The listing builds one solid part. Answer for the finished solid, in the listing's coordinates (mm). Give positions to 0.01 mm unless a question says otherwise; leave off trailing zeros. Order: outer loops, then holes, each group sorted by start corner. A loop starts at its lowest first (then second) coordinate and runs counter-clockwise, first axis right, second up. Notation, with made-up numbers: (1.5, 25.5) - (25.5, 25.5) arc R27 cw to (25.5, 57.5) - close; hole circle Ø7 at (40, -37.5). An arc over 180 degrees is marked (long way). Use CSV: the item, a comma, the result in double quotes.
```python
from build123d import *

# Parameters (mm, degrees)
SKETCH1_W           = 25.4
SKETCH1_H           = 203.2
BOSS_EXTRUDE1_DEPTH = 1.5875


with BuildPart() as part:
    # Sketch1 → Boss-Extrude1 (new body, symmetric)
    with BuildSketch(Plane.XY):
        with Locations((-12.7, -101.6)):
            Rectangle(SKETCH1_W, SKETCH1_H)
        Polygon((152.4, -227.539743973), (152.4, -151.339743973), (0, 0), (0, -203.2), align=None)
    extrude(amount=BOSS_EXTRUDE1_DEPTH, both=True)


solid = part.part
```
Item 1: The part is cut by section A-A (z = -0.95). Give the vertices of the cut face in (x, y), and give its area (3 significant figures).
Taken from the geometry:
outline,"(-25.4, -203.2) - (0, -203.2) - (152.4, -227.54) - (152.4, -151.34) - (0, 0) - (-25.4, 0) - close"
area,"26,500 mm^2"
Item 2: Each of these flat-tipped pins is pushed along its axis until it touches: pin 1 (1.5 mm diameter, centred on x = 118.5, z = 0, fed in from -Y); pin 2 (1.5 mm diameter, centred on y = -56.5, z = -0.5, fed in from +X); pin 3 (1 mm diameter, centred on x = -9, z = 0.5, fed in from -Y). Where does it stop, or does it pass through?
Taken from the geometry:
pin 1,"y = -222.25"
pin 2,"x = 57.65"
pin 3,"y = -203.2"
Item 3: The part is cut by section C-C (y = -77). Give the vertices of the cut face in (x, z), and give its area (3 significant figures).
Taken from the geometry:
outline,"(-25.4, -1.59) - (77.54, -1.59) - (77.54, 1.59) - (-25.4, 1.59) - close"
area,"327 mm^2"
Item 4: Find the intervals of material crossed by line 1 along X through (y, z) = (-15.5, -0.55); line 2 along Y through (x, z) = (130.5, 1.55); line 3 along Y through (x, z) = (87, -0.05), in increasing order.
Taken from the geometry:
line 1,"-25.4 to 15.61"
line 2,"-224.04 to -129.59"
line 3,"-217.09 to -86.39"
Item 5: The part is cut by section B-B (x = 51.5). Give the vertices of the cut face in (y, z).
Taken from the geometry:
outline,"(-211.43, -1.59) - (-51.14, -1.59) - (-51.14, 1.59) - (-211.43, 1.59) - close"
